Autodesk Inventor part; units mm, degrees
ref_plane "YZ Plane" through (0, 0, 0) normal (1, 0, 0) x (0, 1, 0)
ref_plane "XZ Plane" through (0, 0, 0) normal (0, 1, 0) x (-1, 0, 0)
ref_plane "XY Plane" through (0, 0, 0) normal (0, 0, 1) x (1, 0, 0)
sketch "Sketch1" plane through (0, 0, 0) normal (1, 0, 0) x (0, 1, 0)
  line L0 (0, 0) -> (25.4, 0)
  line L1 (25.4, 0) -> (25.4, -25.4)
  line L2 (25.4, -25.4) -> (0, -25.4)
  line L3 (0, -25.4) -> (0, 0)
  line L4 (23.8125, -23.8125) -> (23.8125, -1.5875)
  line L5 (23.8125, -1.5875) -> (1.5875, -1.5875)
  line L6 (1.5875, -1.5875) -> (1.5875, -23.8125)
  line L7 (1.5875, -23.8125) -> (23.8125, -23.8125)
  dimension "d0" = 25.4
  dimension "d1" = 25.4
  dimension "d2" = 1.5875
extrude "Extrusion1" add sketch "Sketch1" along normal blind 304.8
sketch "Sketch2" plane through (0, 25.4, 0) normal (0, 1, 0) x (1, 0, 0)
  line L0 (304.8, 1.5875) -> (304.8, 23.8125)
  line L1 (304.8, 12.7) -> (279.4, 12.7) construction
  circle A0 centre (292.1, 12.7) radius 3.175
  line L2 (304.8, 25.4) -> (304.8, 0)
  circle A1 centre (266.7, 12.7) radius 3.175
  circle A2 centre (63.5, 12.7) radius 3.175
  line L3 (0, 0) -> (0, 25.4)
  dimension "d5" = 6.35
  dimension "d6" = 12.7
  dimension "d9" = 38.1
  dimension "d15" = 63.5
extrude "Extrusion2" cut sketch "Sketch2" against normal blind 25.4
sketch "Sketch3" plane through (0, 0, 0) normal (0, 0, 1) x (1, 0, 0)
  line L0 (0, 0) -> (0, 25.4)
  line L1 (0, 12.7) -> (67.237, 12.7) construction
  circle A0 centre (12.7, 12.7) radius 3.175
  circle A1 centre (38.1, 12.7) radius 3.175
  circle A2 centre (88.9, 12.7) radius 3.175
  dimension "d10" = 6.35
  dimension "d11" = 12.7
  dimension "d12" = 38.1
  dimension "d16" = 88.9
extrude "Extrusion3" cut sketch "Sketch3" against normal blind 88.9
sketch "Sketch4" plane through (0, 25.4, 0) normal (0, 1, 0) x (1, 0, 0)
  point P0 (0, 0)
equation "\"d13\" = d16"
properties part number "Vertical"
Verification items for the finished model (mm, model axes). A direction names the side the tool comes from. Give positions to 0.01 mm unless a question says otherwise; leave off trailing zeros. Order: outer loops, then holes, each group sorted by start corner. A loop starts at its lowest first (then second) coordinate and runs counter-clockwise, first axis right, second up. Notation, with made-up numbers: M 58,30.25 L 70,30.25 A21 cw 70,45.25 Z; hole C 12.5,-31 d3. An arc over 180 degrees is marked long. Answer as a JSON object with one key per item and string values. Group by question number.
1) Mould release check, pull along X, two halves, no side actions. Record for faces 3 (the face through (289.58, 0.8, -10.77)), 4 (the face through (150, 1.588, -13)), 5 (the face through (304.8, 1, -13)): released by +X, released by -X, zero draft, split by the parting line, or undercut.
2) Cross-section at B-B (z = -18.5). Enter the section's corners in (x, y), then the cut area to 3 significant figures.
3) Cross-section at A-A (x = 292.1). Enter the section's corners in (y, z) (1 decimal).
4) Cross-section at C-C (y = 12.7). Give the number of separate pieces and of enclosed holes in the cut face, then the cut area to 3 significant figures.
5) Scan lines: line 1 along X through (y, z) = (0.6, -12.7) (3 decimals); line 2 along Y through (x, z) = (237.5, -16.25); line 3 along Z through (x, y) = (165.5, 2.5). Record each from-to range of solid material in increasing order. Write a range as [from, to].
6) Access from +Z, -Z, +X, -X, +Y, -Y to the whole of each face (thin tool, end or side, straight path). Record for faces 1 (the face through (150, 13, -1.588)), 2 (the face through (66.53, 0.8, -13.65)).
Result sheet:
{
 "1": {"face 3": "undercut", "face 4": "zero draft", "face 5": "released by +X"},
 "2": {"outline": "M 0,0 L 304.8,0 L 304.8,1.59 L 0,1.59 Z; M 0,23.81 L 304.8,23.81 L 304.8,25.4 L 0,25.4 Z", "area": "968 mm2"},
 "3": {"outline": "M 0,-25.4 L 25.4,-25.4 L 25.4,-15.9 L 23.8,-15.9 L 23.8,-23.8 L 1.6,-23.8 L 1.6,-15.9 L 0,-15.9 Z; M 0,-9.5 L 1.6,-9.5 L 1.6,-1.6 L 23.8,-1.6 L 23.8,-9.5 L 25.4,-9.5 L 25.4,0 L 0,0 Z"},
 "4": {"separate pieces": "8", "enclosed holes": "0", "area": "907 mm2"},
 "5": {"line 1": "x = [0, 60.325], [66.675, 263.525], [269.875, 288.925], [295.275, 304.8]", "line 2": "y = [0, 1.59], [23.81, 25.4]", "line 3": "z = [-25.4, -23.81], [-1.59, 0]"},
 "6": {"face 1": "+X, -X", "face 2": "+Y, -Y"}
}
